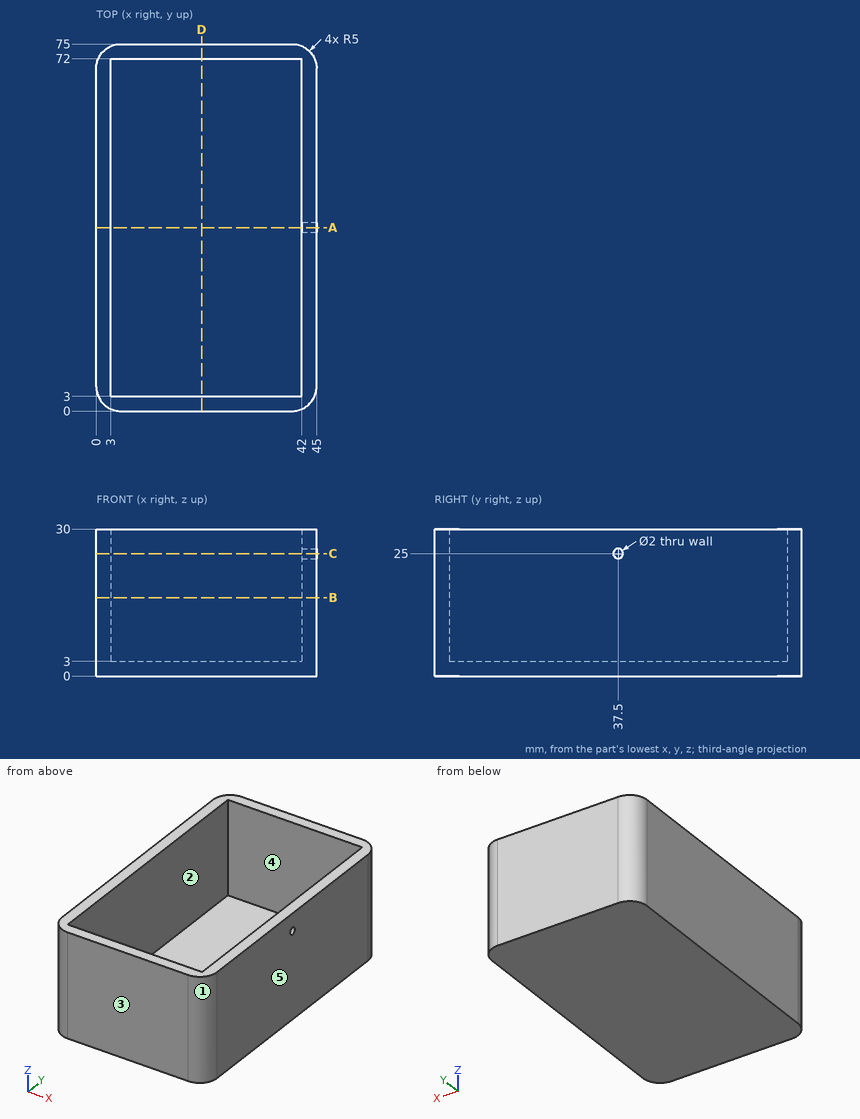
Part print with two shaded views. Sizes in mm from the minimum x, y, z corner. A direction names the side the tool comes from. Round coordinates to 2 decimals unless told otherwise and drop trailing zeros. Order: outer loops, then holes, each group sorted by start corner. A loop starts at its lowest first (then second) coordinate and runs counter-clockwise, first axis right, second up. Notation, with made-up numbers: (21, 47) - (76, 47) arc R4 cw to (76, 54) - close; hole circle Ø7 at (22, -23.5). An arc over 180 degrees is marked (long way). Answer as CSV lines item,"result". Start each with the question number.
1. Saw through at C-C, the plane z = 25. Write the cut outline in (x, y).
2. Pin check, flat tips, straight feed: pin 1 (1.8 mm diameter, centred on y = 37.5, z = 25, fed in from +X); pin 2 (6 mm diameter, centred on x = 23, y = 29.5, fed in from +Z). Stop position of each tip, or through.
3. Saw through at B-B, the plane z = 16. Write the cut outline in (x, y).
4. Tool access for the marked faces 4 and 5: list every direction of +Z, -Z, +X, -X, +Y, -Y with a clear straight run to the whole face (end or side of a thin tool).
5. Saw through at D-D, the plane x = 21.5. Write the cut outline in (y, z).
6. Drill centre lines: L1, parallel to X at y = 47, z = 22.5; L2, parallel to Z at x = 43.55, y = 37.5; L3, parallel to Y at x = 29.5, z = 13.5. Where is each one in solid material? Low to high. Write a range as [from, to].
7. Saw through at A-A, the plane y = 37.5. Write the cut outline in (x, z).
8. Pull direction X, two halves, no side cores. Call the marked faces 1, 2 and 3: +X half, -X half, draft (parallel to the pull), parting line (faces both ways), or undercut.
Model answer:
1,outline,"(0, 5) arc R5 ccw to (5, 0) - (40, 0) arc R5 ccw to (45, 5) - (45, 36.5) - (42, 36.5) - (42, 3) - (3, 3) - (3, 72) - (42, 72) - (42, 38.5) - (45, 38.5) - (45, 70) arc R5 ccw to (40, 75) - (5, 75) arc R5 ccw to (0, 70) - close"
2,pin 1,"stops at x = 3"
2,pin 2,"stops at z = 3"
3,outline,"(0, 5) arc R5 ccw to (5, 0) - (40, 0) arc R5 ccw to (45, 5) - (45, 70) arc R5 ccw to (40, 75) - (5, 75) arc R5 ccw to (0, 70) - close; hole (3, 3) - (42, 3) - (42, 72) - (3, 72) - close"
4,face 4,"+Z"
4,face 5,"+Z, -Z, +X, +Y, -Y"
5,outline,"(0, 0) - (75, 0) - (75, 30) - (72, 30) - (72, 3) - (3, 3) - (3, 30) - (0, 30) - close"
6,L1,"x = [0, 3], [42, 45]"
6,L2,"z = [0, 24], [26, 30]"
6,L3,"y = [0, 3], [72, 75]"
7,outline,"(0, 0) - (45, 0) - (45, 24) - (42, 24) - (42, 3) - (3, 3) - (3, 30) - (0, 30) - close; (42, 26) - (45, 26) - (45, 30) - (42, 30) - close"
8,face 1,"+X half"
8,face 2,"undercut"
8,face 3,"draft"
